from build123d import *

# Parameters (mm, degrees)
SKETCH_1_R                  = 4
EXTRUDE_1_DEPTH             = 37
SKETCH_2_R                  = 4
SKETCH_2_R_2                = 3.9
CUT_EXTRUDE_1_DEPTH         = 1
CUT_EXTRUDE_2_DEPTH         = 38.429934544
CUT_EXTRUDE_2_DEPTH_BACK    = 38.429934544
EXTRUDE_2_REACH             = 39.43
SKETCH_4_R                  = 1.9
EXTRUDE_2_DIRECTION_2_DEPTH = 5


with BuildPart() as part:
    # Sketch 1 → Extrude 1 (new body)
    with BuildSketch(Plane.XY):
        Circle(SKETCH_1_R)
    extrude(amount=EXTRUDE_1_DEPTH)

    # Sketch 2 → Cut-Extrude 1 (cut)
    with BuildSketch(Plane(origin=(0, 0, 0), x_dir=(-1, 0, 0), z_dir=(0, 0, -1))):
        Circle(SKETCH_2_R)
        Circle(SKETCH_2_R_2, mode=Mode.SUBTRACT)
    extrude(amount=-CUT_EXTRUDE_1_DEPTH, mode=Mode.SUBTRACT)

    # Sketch 3 → Cut-Extrude 2 (cut, two sides: drawn at the far end of the back side and taken through both)
    with BuildSketch(Plane(origin=(0, 0, 0), x_dir=(1, 0, 0), z_dir=(0, 1, 0)).offset(-CUT_EXTRUDE_2_DEPTH_BACK)):
        with BuildLine():
            Line((-3, -37), (4, -37))
            Line((4, -37), (4, -34))
            ThreePointArc((4, -34), (0.807886553, -36.218401957), (-3, -37))
        make_face()
    extrude(amount=CUT_EXTRUDE_2_DEPTH + CUT_EXTRUDE_2_DEPTH_BACK, mode=Mode.SUBTRACT)

    # Sketch 4 → Extrude 2 (add, up to next)
    with BuildSketch(Plane.XY.offset(37), mode=Mode.PRIVATE) as extrude_2_sk1:
        with Locations(Location((-2, 0, 0), (0, 0, 238.243136141))):
            Circle(SKETCH_4_R)
    extrude_2_tool1 = extrude(extrude_2_sk1.sketch, amount=-EXTRUDE_2_REACH, mode=Mode.PRIVATE) - part.part
    add(extrude_2_tool1.solids().sort_by_distance((-2, 0, 37))[0])

    # Sketch 4 → Extrude 2 direction 2 (add)
    with BuildSketch(Plane.XY.offset(37)):
        with Locations(Location((-2, 0, 0), (0, 0, 238.243136141))):
            Circle(SKETCH_4_R)
    extrude(amount=EXTRUDE_2_DIRECTION_2_DEPTH)

    # Sketch 5 → Cut-Revolve 3 (revolve, cut)
    with BuildSketch(Plane(origin=(0, 0, 0), x_dir=(0, 0, -1), z_dir=(1, 0, 0))):
        with BuildLine():
            Line((0, 3.5), (0.5, 3.5))
            Line((0.5, 3.5), (0.5, 0))
            Line((0.5, 0), (0, 0))
            ThreePointArc((0, 0), (-0.079251839, 1.256485548), (-0.315751187, 2.493055338))
            ThreePointArc((-0.315751187, 2.493055338), (-0.301514199, 3.041568933), (0, 3.5))
        make_face()
    revolve(axis=Axis((0, 0, 10), (0, 0, -1)), mode=Mode.SUBTRACT)


solid = part.part
Geometry: final body of the model. Coordinates: model frame, mm. A direction names the side the tool comes from. Round coordinates to 2 decimals unless told otherwise and drop trailing zeros. Order: outer loops, then holes, each group sorted by start corner. A loop starts at its lowest first (then second) coordinate and runs counter-clockwise, first axis right, second up. Notation, with made-up numbers: (43.25, 44.5) -> (47.25, 44.5) arc R12 ccw to (47.25, 66.5) -> close; hole circle Ø6 at (36, -38.75). An arc over 180 degrees is marked (long way). Put each result on its own line as item: value. Start each with the question number.
Q1. Line query: probe 1 along Z at (x, y) = (-3, -0.25); probe 2 along X at (y, z) = (0.25, 15); probe 3 along Z at (x, y) = (1, -0.25). Output: solid intervals per line, ascending.
Q2. Section B-B on z = 8.5. Return the cut outline in (x, y).
Q3. First-contact query: pin 1 (3 mm diameter, centred on x = 3, y = 0.5, fed in from +Z); pin 2 (2 mm diameter, centred on y = 1.5, z = 29, fed in from -X). Flat tips, straight axial feed; report the tip coordinate or a pass-through.
Q4. Reachability of faces 1 (the cylindrical face through (-4, 0, 19)), 2 (the cylindrical face through (-0.17, 0.51, 39.24)), 3 (the cylindrical face through (2.87, 2.64, 0.49)) from +Z, -Z, +X, -X, +Y, -Y: full face, straight path, thin tool, end or side. Return the list, or none.
Q5. Section A-A on y = 0. Return the cut outline in (x, z), and give its area (3 significant figures).
Ans:
1. probe 1: z = 0.31 to 42
1. probe 2: x = -3.99 to 3.99
1. probe 3: z = 0.05 to 36.13
2. outline: circle Ø8 at (0, 0)
3. pin 1: stops at z = 35.89
3. pin 2: stops at x = -3.97
4. face 1: +Z, -Z
4. face 2: +Z
4. face 3: -Z
5. outline: (-4, 1) -> (-3.9, 1) -> (-3.9, 0) -> (-3.5, 0) arc R1 cw to (-2.49, 0.32) arc R10 ccw to (2.49, 0.32) arc R1 cw to (3.5, 0) -> (3.9, 0) -> (3.9, 1) -> (4, 1) -> (4, 34) arc R9.67 ccw to (-0.1, 36.55) -> (-0.1, 42) -> (-3.9, 42) -> (-3.9, 37) -> (-4, 37) -> close
5. area: 308 mm2
